Autodesk Inventor part; units mm, degrees
ref_plane "YZ Plane" through (0, 0, 0) normal (1, 0, 0) x (0, 1, 0)
ref_plane "XZ Plane" through (0, 0, 0) normal (0, 1, 0) x (-1, 0, 0)
ref_plane "XY Plane" through (0, 0, 0) normal (0, 0, 1) x (1, 0, 0)
sketch "Sketch1" plane through (0, 0, 0) normal (0, 1, 0) x (-1, 0, 0)
  line L0 (75, 33.3333) -> (-75, 33.3333)
  line L1 (-75, 33.3333) -> (-75, -66.6667)
  line L2 (-75, -66.6667) -> (75, -66.6667)
  line L3 (75, -66.6667) -> (75, 33.3333)
  point P0 (0, 0)
  dimension "d0" = 100
  dimension "d1" = 150
extrude "Extrusion1" add sketch "Sketch1" along normal blind 47
sketch "Sketch2" plane through (75, 0, 33.3333) normal (1, 0, 0) x (0, 0, -1)
  line L0 (15, -11) -> (85, -11)
  line L1 (85, -11) -> (85, 32)
  line L2 (85, 32) -> (15, 32)
  line L3 (15, 32) -> (15, -11)
  line L4 (0, 47) -> (100, 47)
  line L5 (100, 0) -> (100, 47)
  line L6 (0, 0) -> (0, 47)
  point P0 (33.3333, 0)
  dimension "d4" = 15
  dimension "d5" = 15
  dimension "d6" = 15
extrude "Extrusion2" cut sketch "Sketch2" against normal blind 200
sketch "Sketch3" plane through (75, 0, -66.6667) normal (1, 0, 0) x (0, 0, -1)
  line L0 (-100, 0) -> (-100, 47)
  line L1 (-100, 0) -> (-112.5, 0)
  line L2 (-112.5, 0) -> (-112.5, 15)
  line L3 (-112.5, 15) -> (-100, 15)
  line L4 (-100, 15) -> (-100, 0)
  line L5 (0, 0) -> (0, 47)
  line L6 (0, 0) -> (12.5, 0)
  line L7 (12.5, 0) -> (12.5, 15)
  line L8 (12.5, 15) -> (0, 15)
  line L9 (0, 15) -> (0, 0)
  point P0 (-66.6667, 0)
  point P1 (0, 15)
  dimension "d9" = 12.5
  dimension "d10" = 12.5
  dimension "d11" = 15
  dimension "d12" = 15
extrude "Extrusion3" add sketch "Sketch3" against normal blind 160
properties part number "ZadBabkaPodkladka" material "Aluminum 6061-AHC"
Here's how the part is built. I have some questions about the finished solid (model axes, mm). A direction names the side the tool comes from. Coordinates: 2 decimals unless noted, no trailing zeros. Write each loop counter-clockwise with the first axis right and the second up, starting at its lowest first coordinate (ties: lowest second). Pieces come first, ordered by that corner, then holes. Notation, with made-up numbers: (-24, 44.25) -> (13, 44.25) arc R20 cw to (13, 56.25) -> close; hole circle Ø2 at (68.5, -29). An arc over 180 degrees is marked (long way). Use a Markdown table: item, result. Add a question column.
(1) I'm going to push flat-ended pins straight in: P1, Ø12, axis at x = -22.5, y = 30, coming from the +Z side; P2, Ø4, axis at x = 4, z = -24, coming from the -Y side; P3, Ø23.5, axis at y = 26, z = -6.5, coming from the -X side. Where does each tip first touch, or does it pass through?
(2) If we section it at B-B, the plane x = -70: Write out the boundary of the cut face in (y, z).
(3) If we section it at A-A, the plane y = 19: Write out the boundary of the cut face in (x, z), and give its area (3 significant figures).
(4) If we section it at C-C, the plane z = 23.5: Write out the boundary of the cut face in (x, y), and give its area (3 significant figures).
(5) If we section it at D-D, the plane y = 38: Write out the boundary of the cut face in (x, z), and give its area (3 significant figures).
(6) For faces 1 (the flat face through (-80, 7, 33.333)), 2 (the flat face through (-4, 15, 40)), 3 (the flat face through (1, 16, -51.667)), which set-ups out of +Z, -Z, +X, -X, +Y, -Y let a thin tool reach every point of the face, with its end or its side?
(7) We'd pull the mould along Z, two halves only. Please class faces 4 (the flat face through (75, 34, -16)), 5 (the flat face through (-75, 34, -17)), 6 (the flat face through (-4, 7, 45.833)): +Z half, -Z half, draft (parallel to the pull), parting line (faces both ways), or undercut.
(8) Please list where these lines run through material, in increasing order: line 1 (Z direction, x = -50.5, y = 26.5); line 2 (Z direction, x = -73.5, y = 8.5); line 3 (X direction, y = 8, z = -52).
Outcome:
| question | item | result |
|---|---|---|
| 1 | P1 | stops at z = 33.33 |
| 1 | P2 | stops at y = 32 |
| 1 | P3 | stops at x = -75 |
| 2 | outline | (0, -79.17) -> (15, -79.17) -> (15, -66.67) -> (47, -66.67) -> (47, 33.33) -> (15, 33.33) -> (15, 45.83) -> (0, 45.83) -> (0, 18.33) -> (32, 18.33) -> (32, -51.67) -> (0, -51.67) -> close |
| 3 | outline | (-75, -66.67) -> (75, -66.67) -> (75, -51.67) -> (-75, -51.67) -> close; (-75, 18.33) -> (75, 18.33) -> (75, 33.33) -> (-75, 33.33) -> close |
| 3 | area | 4,500 mm^2 |
| 4 | outline | (-75, 0) -> (75, 0) -> (75, 47) -> (-75, 47) -> close |
| 4 | area | 7,050 mm^2 |
| 5 | outline | (-75, -66.67) -> (75, -66.67) -> (75, 33.33) -> (-75, 33.33) -> close |
| 5 | area | 15,000 mm^2 |
| 6 | face 1 | -X, +Y, -Y |
| 6 | face 2 | +Z, +X, -X, +Y |
| 6 | face 3 | +X, -X, -Y |
| 7 | face 4 | draft |
| 7 | face 5 | undercut |
| 7 | face 6 | +Z half |
| 8 | line 1 | z = -66.67 to -51.67, 18.33 to 33.33 |
| 8 | line 2 | z = -79.17 to -51.67, 18.33 to 45.83 |
| 8 | line 3 | x = -75 to 75 |
